```python
from build123d import *

# Parameters (mm, degrees)
SKETCH1_W           = 67
SKETCH1_H           = 57
SKETCH1_R           = 1.55
BOSS_EXTRUDE1_DEPTH = 4
SKETCH2_R           = 1.05
CUT_EXTRUDE1_DEPTH  = 45.164465354
CHAMFER1_SIZE       = 2


with BuildPart() as part:
    # Sketch1 → Boss-Extrude1 (new body)
    with BuildSketch(Plane(origin=(0, 0, 0), x_dir=(1, 0, 0), z_dir=(0, 1, 0))):
        Rectangle(SKETCH1_W, SKETCH1_H)
        with Locations(Location((15, 8.25, 0), (0, 0, 270))):
            Circle(SKETCH1_R, mode=Mode.SUBTRACT)
        with Locations(Location((-15, 8.25, 0), (0, 0, 90))):
            Circle(SKETCH1_R, mode=Mode.SUBTRACT)
        with Locations(Location((-15, -8.25, 0), (0, 0, 270))):
            Circle(SKETCH1_R, mode=Mode.SUBTRACT)
        with Locations(Location((15, -8.25, 0), (0, 0, 90))):
            Circle(SKETCH1_R, mode=Mode.SUBTRACT)
    extrude(amount=BOSS_EXTRUDE1_DEPTH)

    # Sketch2 → Cut-Extrude1 (cut, through all)
    with BuildSketch(Plane(origin=(0, 4, 0), x_dir=(1, 0, 0), z_dir=(0, 1, 0))):
        with Locations(Location((29, 24.5, 0), (0, 0, 270))):
            Circle(SKETCH2_R)
        with Locations(Location((-29, 24.5, 0), (0, 0, 90))):
            Circle(SKETCH2_R)
        with Locations(Location((-29, -24.5, 0), (0, 0, 270))):
            Circle(SKETCH2_R)
        with Locations(Location((29, -24.5, 0), (0, 0, 90))):
            Circle(SKETCH2_R)
    extrude(amount=-CUT_EXTRUDE1_DEPTH, mode=Mode.SUBTRACT)

    # Chamfer1
    chamfer1_edges = [part.edges().sort_by_distance(p)[0] for p in [
        (33.5, 2, 28.5),
        (-33.5, 2, 28.5),
        (-33.5, 2, -28.5),
        (33.5, 2, -28.5),
    ]]
    chamfer(chamfer1_edges, length=CHAMFER1_SIZE)


solid = part.part
```
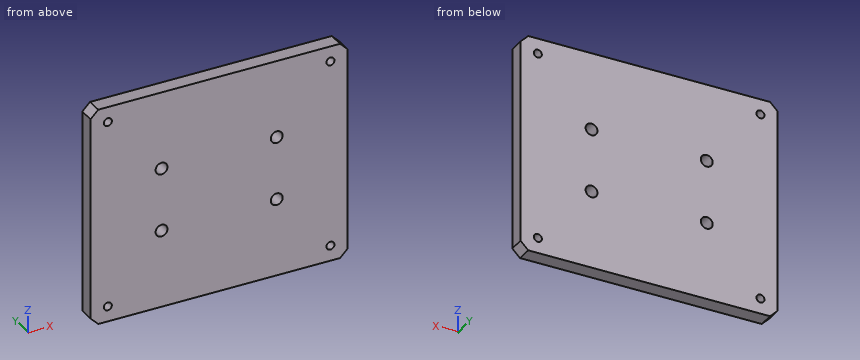
Design review of the part built by this model. Coordinates are the model's own, in mm. Give positions to 0.01 mm unless a question says otherwise; leave off trailing zeros. Write each loop counter-clockwise with the first axis right and the second up, starting at its lowest first coordinate (ties: lowest second). Pieces come first, ordered by that corner, then holes.
(1) Wall thickness on line 1 along X through (y, z) = (2.65, 24.5); line 2 along X through (y, z) = (2.55, 8.25); line 3 along Z through (x, y) = (-28.5, 3.6): over which ranges is each line inside the solid? List them lowest first.
Checked values:
line 1: x = -33.5 to -30.05, -27.95 to 27.95, 30.05 to 33.5
line 2: x = -33.5 to -16.55, -13.45 to 13.45, 16.55 to 33.5
line 3: z = -28.5 to -25.42, -23.58 to 23.58, 25.42 to 28.5
(2) Add section B-B (x = 29). Give the boundary of the cut face in (y, z).
Checked values:
outline: (0, -28.5) - (4, -28.5) - (4, -25.55) - (0, -25.55) - close; (0, -23.45) - (4, -23.45) - (4, 23.45) - (0, 23.45) - close; (0, 25.55) - (4, 25.55) - (4, 28.5) - (0, 28.5) - close
(3) Add section A-A (z = 24.5). Give the boundary of the cut face in (x, y).
Checked values:
outline: (-33.5, 0) - (-30.05, 0) - (-30.05, 4) - (-33.5, 4) - close; (-27.95, 0) - (27.95, 0) - (27.95, 4) - (-27.95, 4) - close; (30.05, 0) - (33.5, 0) - (33.5, 4) - (30.05, 4) - close
(4) Clearance check with a flat-ended pin moving along its axis: pin 1 Ø2.5 at (x, z) = (-15, -8.25) entering from +Y. State where the tip first meets the part, or that it passes through.
Checked values:
pin 1: passes through
